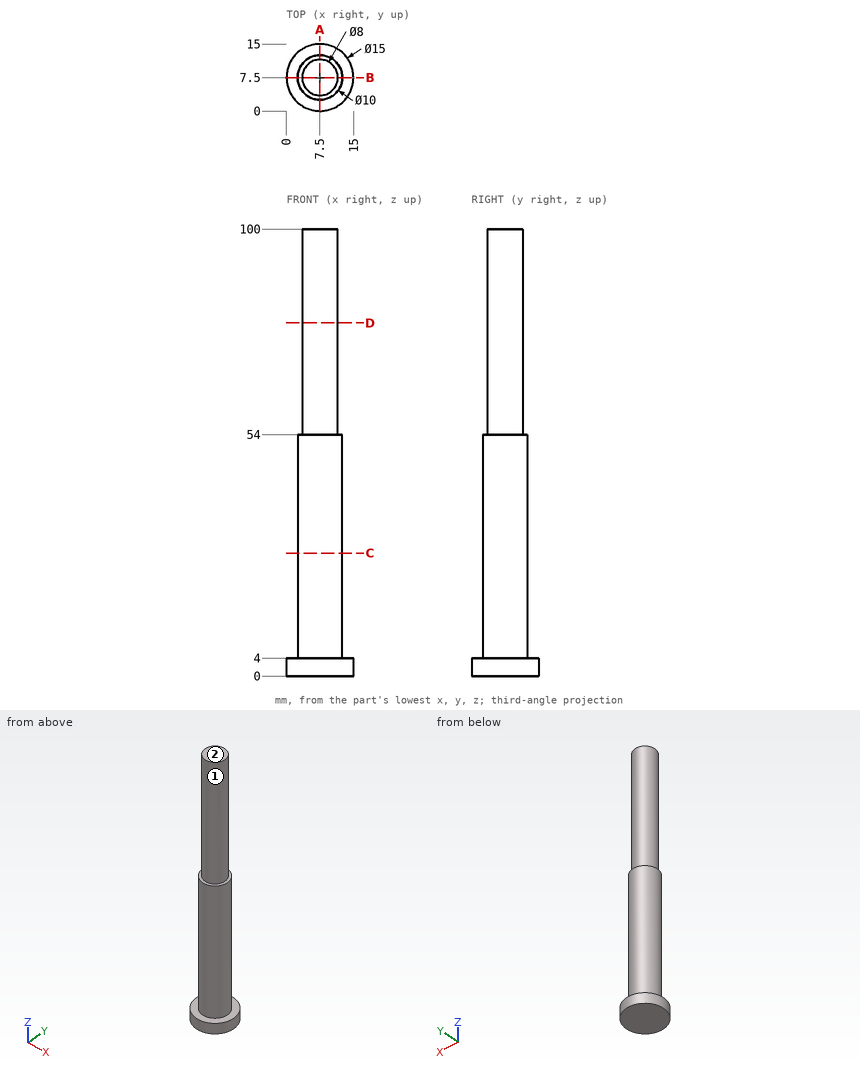
Geometry check sheet. Reference: drawing and pictorial views, mm from the part's lowest x, y, z. A direction names the side the tool comes from. Give positions to 0.01 mm unless a question says otherwise; leave off trailing zeros. Order: outer loops, then holes, each group sorted by start corner. A loop starts at its lowest first (then second) coordinate and runs counter-clockwise, first axis right, second up. Notation, with made-up numbers: M -37.75,60.5 L 8.25,60.5 A33 ccw 8.25,93.5 Z; hole C 61,19 d5. An arc over 180 degrees is marked long. Return JSON: item names as keys, results as strings. Group by question number.
1) Section check C-C on z = 27.5. Record the cut outline in (x, y).
2) Scan lines: line 1 (Z direction, x = 11.5, y = 13.5); line 2 (Y direction, x = 7.5, z = 36.5); line 3 (X direction, y = 4.5, z = 17). Record each from-to range of solid material in increasing order.
3) Go/stop test with flat-tipped pins: pin 1 Ø4.5 at (x, y) = (11, 10.5) entering from +Z; pin 2 Ø5 at (y, z) = (13.5, 55) entering from +X; pin 3 Ø8 at (y, z) = (8, 53.5) entering from -X; pin 4 Ø1.5 at (y, z) = (6, 65.5) entering from +X. Record where each tip stops, or that it passes through.
4) Section check D-D on z = 79. Record the cut outline in (x, y), and give its area (3 significant figures).
5) Section check A-A on x = 7.5. Record the cut outline in (y, z), and give its area (3 significant figures).
6) Access from +Z, -Z, +X, -X, +Y, -Y to the whole of each face (thin tool, end or side, straight path). Record for the marked faces 1 and 2.
Answer block:
{
 "1": {"outline": "C 7.5,7.5 d10"},
 "2": {"line 1": "z = 0 to 4", "line 2": "y = 2.5 to 12.5", "line 3": "x = 3.5 to 11.5"},
 "3": {"pin 1": "stops at z = 100", "pin 2": "stops at x = 10.85", "pin 3": "stops at x = 2.5", "pin 4": "stops at x = 11.43"},
 "4": {"outline": "C 7.5,7.5 d8", "area": "50.3 mm^2"},
 "5": {"outline": "M 0,0 L 15,0 L 15,4 L 12.5,4 L 12.5,54 L 11.5,54 L 11.5,100 L 3.5,100 L 3.5,54 L 2.5,54 L 2.5,4 L 0,4 Z", "area": "928 mm^2"},
 "6": {"face 1": "+Z", "face 2": "+Z, +X, -X, +Y, -Y"}
}
